The listing builds one solid part. Answer for the finished solid, in the listing's coordinates (mm). Face numbers are marked on the shaded views. Round coordinates to 2 decimals unless told otherwise and drop trailing zeros. Order: outer loops, then holes, each group sorted by start corner. A loop starts at its lowest first (then second) coordinate and runs counter-clockwise, first axis right, second up. Notation, with made-up numbers: (75.5, -26.75) - (113.5, -26.75) arc R16 cw to (113.5, -11.75) - close; hole circle Ø3 at (77.25, 48). An arc over 180 degrees is marked (long way). Use CSV: the item, a comma, the result in double quotes. Start each with the question number.
Item 1: Determine the mould class of the marked faces 1, 2 and 3 for opening direction Y: +Y half, -Y half, draft (parallel to the pull), parting line (faces both ways), or undercut.
Item 2: Straight lines are drawn through the part: line 1 along Z through (x, y) = (0.5, -1.75); line 2 along Y through (x, z) = (1, 0.1); line 3 along Y through (x, z) = (0.1, 0.4). For each, find the intervals that lie inside material, in ascending order. Write a range as [from, to].
Item 3: Find section A-A, the plane x = 0.1. Give the vertices of the cut face in (y, z).
Item 4: Find section B-B, the plane y = -1.5. Give the vertices of the cut face in (x, z), plus the area to 3 significant figures.
Item 5: A flat-ended cylindrical pin translates along its axis: P1, Ø0.7, axis at x = 0.5, y = 0, coming from the +Z side. Find the tip coordinate at first contact, or state that the pin passes through.
Autodesk Inventor part; units mm, degrees
ref_plane "YZ Plane" through (0, 0, 0) normal (1, 0, 0) x (0, 1, 0)
ref_plane "XZ Plane" through (0, 0, 0) normal (0, 1, 0) x (-1, 0, 0)
ref_plane "XY Plane" through (0, 0, 0) normal (0, 0, 1) x (1, 0, 0)
sketch "Sketch1" plane through (0, 0, 0) normal (1, 0, 0) x (0, 1, 0)
  line L0 (-6.5, 0) -> (3.5, 0)
  line L1 (-6.5, 0) -> (-6.5, 0.3)
  line L2 (-6.5, 0.3) -> (3.337, 0.3)
  line L3 (5.5, 0) -> (5.6721, 0.2457)
  line L4 (5.6721, 0.2457) -> (5.1721, 0.5958)
  line L5 (5.5, 0) -> (5, 0.3501)
  arc A0 (5, 0.3501) -> (3.5, 0) centre (4.4069, -0.497) ccw
  arc A1 (5.1721, 0.5958) -> (3.337, 0.3) centre (4.4069, -0.497) ccw
  point P0 (0, 0)
  dimension "d0" = 0.3
  dimension "d3" = 6.5
  dimension "d4" = 10
  dimension "d5" = 35
  dimension "d6" = 2
  dimension "d7" = 0.3
  dimension "d8" = 1.5
extrude "Extrusion1" add sketch "Sketch1" along normal blind 1.35
fillet "Fillet1" radius 0.75 1 edges at (0.675, 3.337, 0.3)
fillet "Fillet2" radius 0.75 1 edges at (0.675, 3.5, 0)
equation "\"d7\" = d0"
properties material "Bronze, Soft Tin"
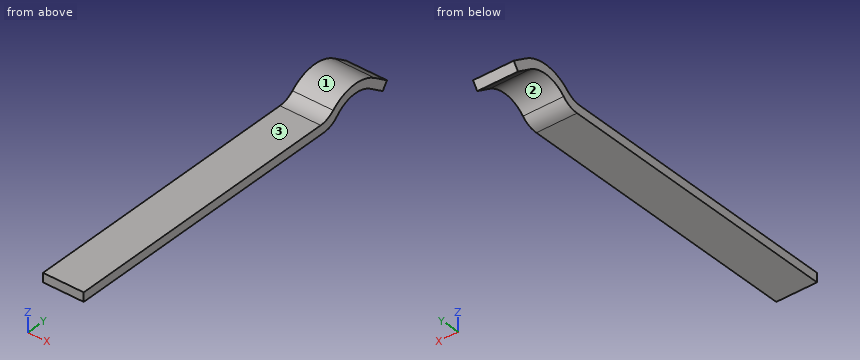
Worked out:
1,face 1,"parting line"
1,face 2,"undercut"
1,face 3,"draft"
2,line 1,"z = [0, 0.3]"
2,line 2,"y = [-6.5, 3.51], [5.36, 5.57]"
2,line 3,"y = [3.38, 3.89], [4.92, 5.45]"
3,outline,"(-6.5, 0) - (3.13, 0) arc R0.75 ccw to (3.67, 0.23) arc R1.03 cw to (5, 0.35) - (5.5, 0) - (5.67, 0.25) - (5.17, 0.6) arc R1.33 ccw to (3.51, 0.49) arc R0.75 cw to (3.01, 0.3) - (-6.5, 0.3) - close"
4,outline,"(0, 0) - (1.35, 0) - (1.35, 0.3) - (0, 0.3) - close"
4,area,"0.405 mm²"
5,P1,"stops at z = 0.3"
